```python
from build123d import *

# Parameters (mm, degrees)
F1_W          = 38.4
F1_H          = 38.4
F1_W_2        = 36.4
F1_H_2        = 36.4
F2_DEPTH      = 4.8
F3_R          = 1.5
F3_W          = 38.4
F3_H          = 38.4
F3_W_2        = 36.4
F3_H_2        = 36.4
F4_DEPTH      = 2
F4_DEPTH_BACK = 1
F5_R          = 0.6
F6_W          = 8
F6_H          = 1
F7_DEPTH      = 0.5


with BuildPart() as f2:
    # F1 (on Top) → F2 (new body)
    with BuildSketch(Plane.XY):
        Rectangle(F1_W, F1_H)
        Rectangle(F1_W_2, F1_H_2, mode=Mode.SUBTRACT)
    extrude(amount=F2_DEPTH)

    # F3 (on face) → F4 (join, two sides)
    with BuildSketch(Plane.XY.offset(4.8)) as f4_sk:
        with BuildLine():
            ThreePointArc((-35, -46.5), (-34.12132, -48.62132), (-32, -49.5))
            Line((-32, -49.5), (-22, -49.5))
            ThreePointArc((-22, -49.5), (-19.87868, -48.62132), (-19, -46.5))
            Line((-19, -46.5), (-19, -45.438493))
            ThreePointArc((-19, -45.438493), (-18.950318, -44.894781), (-18.802918, -44.369078))
            Line((-18.802918, -44.369078), (-13.230511, -29.763898))
            ThreePointArc((-13.230511, -29.763898), (-12.151972, -28.06913), (-10.493455, -26.935637))
            Line((-10.493455, -26.935637), (-3.057386, -23.81569))
            ThreePointArc((-3.057386, -23.81569), (0.049323, -23.192689), (3.154219, -23.824657))
            Line((3.154219, -23.824657), (10.503716, -26.933267))
            ThreePointArc((10.503716, -26.933267), (12.153945, -28.066345), (13.227468, -29.755923))
            Line((13.227468, -29.755923), (18.802918, -44.369078))
            ThreePointArc((18.802918, -44.369078), (18.950318, -44.894781), (19, -45.438493))
            Line((19, -45.438493), (19, -46.5))
            ThreePointArc((19, -46.5), (19.87868, -48.62132), (22, -49.5))
            Line((22, -49.5), (32, -49.5))
            ThreePointArc((32, -49.5), (34.12132, -48.62132), (35, -46.5))
            Line((35, -46.5), (35, -44.801084))
            ThreePointArc((35, -44.801084), (34.484786, -43.120061), (33.116107, -42.016429))
            ThreePointArc((33.116107, -42.016429), (31.618403, -41.017341), (30.649398, -39.5))
            Line((30.649398, -39.5), (26.524716, -28.620354))
            ThreePointArc((26.524716, -28.620354), (26.281849, -27.748859), (26.2, -26.847865))
            Line((26.2, -26.847865), (26.2, 11.797695))
            ThreePointArc((26.2, 11.797695), (27.038254, 14.568952), (29.271947, 16.411003))
            Line((29.271947, 16.411003), (33.054434, 17.991828))
            ThreePointArc((33.054434, 17.991828), (34.344715, 19.024405), (34.892422, 20.58359))
            Line((34.892422, 20.58359), (34.99482, 22.323777))
            ThreePointArc((34.99482, 22.323777), (34.18231, 24.558524), (31.99876, 25.5))
            Line((31.99876, 25.5), (21.997216, 25.495866))
            ThreePointArc((21.997216, 25.495866), (20.678268, 25.189768), (19.628246, 24.334917))
            ThreePointArc((19.628246, 24.334917), (17.87728, 22.90971), (15.677896, 22.4))
            Line((15.677896, 22.4), (-15.677896, 22.4))
            ThreePointArc((-15.677896, 22.4), (-17.87728, 22.90971), (-19.628246, 24.334917))
            ThreePointArc((-19.628246, 24.334917), (-20.678268, 25.189768), (-21.997216, 25.495866))
            Line((-21.997216, 25.495866), (-31.99876, 25.5))
            ThreePointArc((-31.99876, 25.5), (-34.18231, 24.558524), (-34.99482, 22.323777))
            Line((-34.99482, 22.323777), (-34.892422, 20.58359))
            ThreePointArc((-34.892422, 20.58359), (-34.344715, 19.024405), (-33.054434, 17.991828))
            Line((-33.054434, 17.991828), (-29.271947, 16.411003))
            ThreePointArc((-29.271947, 16.411003), (-27.038254, 14.568952), (-26.2, 11.797695))
            Line((-26.2, 11.797695), (-26.2, -26.847865))
            ThreePointArc((-26.2, -26.847865), (-26.281849, -27.748859), (-26.524716, -28.620354))
            Line((-26.524716, -28.620354), (-30.649398, -39.5))
            ThreePointArc((-30.649398, -39.5), (-31.618403, -41.017341), (-33.116107, -42.016429))
            ThreePointArc((-33.116107, -42.016429), (-34.484786, -43.120061), (-35, -44.801084))
            Line((-35, -44.801084), (-35, -46.5))
        make_face()
        with Locations((-32, -46.5)):
            Circle(F3_R, mode=Mode.SUBTRACT)
        with Locations((-22, -46.5)):
            Circle(F3_R, mode=Mode.SUBTRACT)
        with Locations((22, -46.5)):
            Circle(F3_R, mode=Mode.SUBTRACT)
        with Locations((32, -46.5)):
            Circle(F3_R, mode=Mode.SUBTRACT)
        with BuildLine():
            ThreePointArc((-20.5, -17.5), (-22, -19), (-23.5, -17.5))
            Line((-23.5, -17.5), (-23.5, 17.5))
            ThreePointArc((-23.5, 17.5), (-22, 19), (-20.5, 17.5))
            Line((-20.5, 17.5), (-20.5, -17.5))
        make_face(mode=Mode.SUBTRACT)
        with Locations((-32, 22.5)):
            Circle(F3_R, mode=Mode.SUBTRACT)
        with Locations((-21.998456, 22.495866)):
            Circle(F3_R, mode=Mode.SUBTRACT)
        Rectangle(F3_W, F3_H, mode=Mode.SUBTRACT)
        with BuildLine():
            ThreePointArc((20.5, 17.5), (22, 19), (23.5, 17.5))
            Line((23.5, 17.5), (23.5, -17.5))
            ThreePointArc((23.5, -17.5), (22, -19), (20.5, -17.5))
            Line((20.5, -17.5), (20.5, 17.5))
        make_face(mode=Mode.SUBTRACT)
        with Locations((22, 22.5)):
            Circle(F3_R, mode=Mode.SUBTRACT)
        with Locations((32, 22.5)):
            Circle(F3_R, mode=Mode.SUBTRACT)
        Rectangle(F3_W, F3_H)
        Rectangle(F3_W_2, F3_H_2, mode=Mode.SUBTRACT)
    extrude(amount=F4_DEPTH)
    extrude(f4_sk.sketch, amount=-F4_DEPTH_BACK)

    # F5
    f5_edges = [f2.edges().sort_by_distance(p)[0] for p in [
        (-19.2, -19.2, 1.9),
        (19.2, -19.2, 1.9),
        (19.2, 19.2, 1.9),
        (-19.2, 19.2, 1.9),
    ]]
    fillet(f5_edges, radius=F5_R)

    # F6 (on face) → F7 (cut)
    with BuildSketch(Plane.XY.offset(6.8)):
        with Locations((-22.2, 0)):
            Rectangle(F6_W, F6_H)
        with Locations((22.2, 0)):
            Rectangle(F6_W, F6_H)
    extrude(amount=-F7_DEPTH, mode=Mode.SUBTRACT)


solid = f2.part
```
Source: CAD feature listing. Evaluate the final solid. Frame: model axes, mm. A direction names the side the tool comes from. Coordinates: 2 decimals unless noted, no trailing zeros. Loops run counter-clockwise (first coordinate to the right, second up) from the corner with the lowest first, then second, coordinate; pieces in that order, holes last. Notation, with made-up numbers: M 26,72 L 45,72 A35 ccw 45,106 Z; hole C 87.5,73 d10. An arc over 180 degrees is marked long. Use a Markdown table: item, result. Add a question column.
Q1. Draft query along Y for faces 5 (the cylindrical face through (34.5, -43.14, 5.32)), 6 (the flat face through (35, -46, 5)), 7 (the cylindrical face through (-26.28, -27.74, 5.32)), 8 (the flat face through (0, 19.2, 2)). Return one class per face: pulls with the +Y half, pulls with the -Y half, needs draft (parallel to the pull), parting line crosses it, or undercut.
Q2. Material intervals for L1, parallel to X at y = -2.5, z = 6.5; L2, parallel to Y at x = -22, z = 6.3; L3, parallel to Y at x = 9.5, z = 1.5, sorted ascending.
Q3. Section query C-C, the plane x = -1.5. Return loops of the section in (y, z), and give its area (3 significant figures).
Q4. First-contact query: pin 1 (2.5 mm diameter, centred on x = 22, y = -46.5, fed in from +Z) (1 decimal); pin 2 (5 mm diameter, centred on x = 22.5, y = -25.5, fed in from -Z); pin 3 (0.8 mm diameter, centred on x = 19, y = 0, fed in from +Z); pin 4 (3.5 mm diameter, centred on x = -7.5, z = 3.5, fed in from +Y). Flat tips, straight axial feed; report the tip coordinate or a pass-through.
Q5. Access query for faces 1 (the cylindrical face through (-20.7, 25.2, 5.3)), 2 (the cylindrical face through (26.284, -27.761, 5.321)), 3 (the cylindrical face through (-34.358, 19.044, 5.321)), 4 (the flat face through (6.78, -25.36, 5.32)). Directions: +Z, -Z, +X, -X, +Y, -Y. A direction counts if a zero-diameter tool reaches every point of the face in a straight line with its end or side. Return the directions, or none.
Q6. Section query D-D, the plane y = -41. Return loops of the section in (x, z), and give its area (3 significant figures).
Q7. Section query A-A, the plane y = 6. Return loops of the section in (x, z), and give its area (3 significant figures).
Q8. Section query B-B, the plane z = 2.25. Return loops of the section in (x, y).
Result:
| question | item | result |
|---|---|---|
| 1 | face 5 | undercut |
| 1 | face 6 | needs draft |
| 1 | face 7 | undercut |
| 1 | face 8 | pulls with the +Y half |
| 2 | L1 | x = -26.2 to -23.5, -20.5 to -18.2, 18.2 to 20.5, 23.5 to 26.2 |
| 2 | L2 | y = -49.5 to -48, -45 to -19, 19 to 21, 24 to 25.5 |
| 2 | L3 | y = -19.2 to -18.2, 18.2 to 19.2 |
| 3 | outline | M -23.34,3.8 L -19.2,3.8 L -19.2,0 L -18.2,0 L -18.2,6.8 L -23.34,6.8 Z; M 18.2,0 L 19.2,0 L 19.2,3.8 L 22.4,3.8 L 22.4,6.8 L 18.2,6.8 Z |
| 3 | area | 35.6 mm2 |
| 4 | pin 1 | passes through |
| 4 | pin 2 | stops at z = 3.8 |
| 4 | pin 3 | stops at z = 6.3 |
| 4 | pin 4 | stops at y = 22.4 |
| 5 | face 1 | +Z, -Z, +Y |
| 5 | face 2 | +Z, -Z, +X |
| 5 | face 3 | +Z, -Z, -X |
| 5 | face 4 | +Z, -Z, -Y |
| 6 | outline | M -31.6,3.8 L -17.52,3.8 L -17.52,6.8 L -31.6,6.8 Z; M 17.52,3.8 L 31.6,3.8 L 31.6,6.8 L 17.52,6.8 Z |
| 6 | area | 84.5 mm2 |
| 7 | outline | M -26.2,3.8 L -23.5,3.8 L -23.5,6.8 L -26.2,6.8 Z; M -20.5,3.8 L -19.2,3.8 L -19.2,0 L -18.2,0 L -18.2,6.8 L -20.5,6.8 Z; M 18.2,0 L 19.2,0 L 19.2,3.8 L 20.5,3.8 L 20.5,6.8 L 18.2,6.8 Z; M 23.5,3.8 L 26.2,3.8 L 26.2,6.8 L 23.5,6.8 Z |
| 7 | area | 37.6 mm2 |
| 8 | outline | M -19.2,-18.6 A0.6 ccw -18.6,-19.2 L 18.6,-19.2 A0.6 ccw 19.2,-18.6 L 19.2,18.6 A0.6 ccw 18.6,19.2 L -18.6,19.2 A0.6 ccw -19.2,18.6 Z; hole M -18.2,-18.2 L 18.2,-18.2 L 18.2,18.2 L -18.2,18.2 Z |
